Geometry: see drawing. Coordinates: mm, zero at the bounding-box minimum. A direction names the side the tool comes from. Coordinates: 2 decimals unless noted, no trailing zeros. Write each loop counter-clockwise with the first axis right and the second up, starting at its lowest first coordinate (ties: lowest second). Pieces come first, ordered by that corner, then holes.
1) Section query C-C (y = 4). Output: boundary loops of the cut face in (x, z), then the cut area to 3 significant figures.
2) Pin query (flat end, axial travel): pin 1 Ø3 at (x, z) = (13, 1) entering from +Y; pin 2 Ø4 at (x, z) = (36.5, 7) entering from +Y (1 decimal); pin 3 Ø3 at (x, z) = (33.5, 5) entering from -Y; pin 4 Ø1 at (y, z) = (43.5, 5) entering from +X (1 decimal). Return the tip coordinate at first contact, or that it passes through.
3) Section query B-B (z = 6). Output: boundary loops of the cut face in (x, y) (1 decimal).
4) Section query D-D (z = 2). Output: boundary loops of the cut face in (x, y).
5) Line query: L1, parallel to Y at x = 50, z = 7.75 (1 decimal); L2, parallel to X at y = 7.5, z = 7.25 (1 decimal); L3, parallel to Z at x = 31, y = 23.5. Output: solid intervals per line, ascending.
6) Section query A-A (x = 5). Output: boundary loops of the cut face in (y, z).
7) Set-up query: the marked faces 1 and 2. Return all of +Z, -Z, +X, -X, +Y, -Y with unobstructed straight access to the full face (end or side cutting, diameter ignored); none if empty.
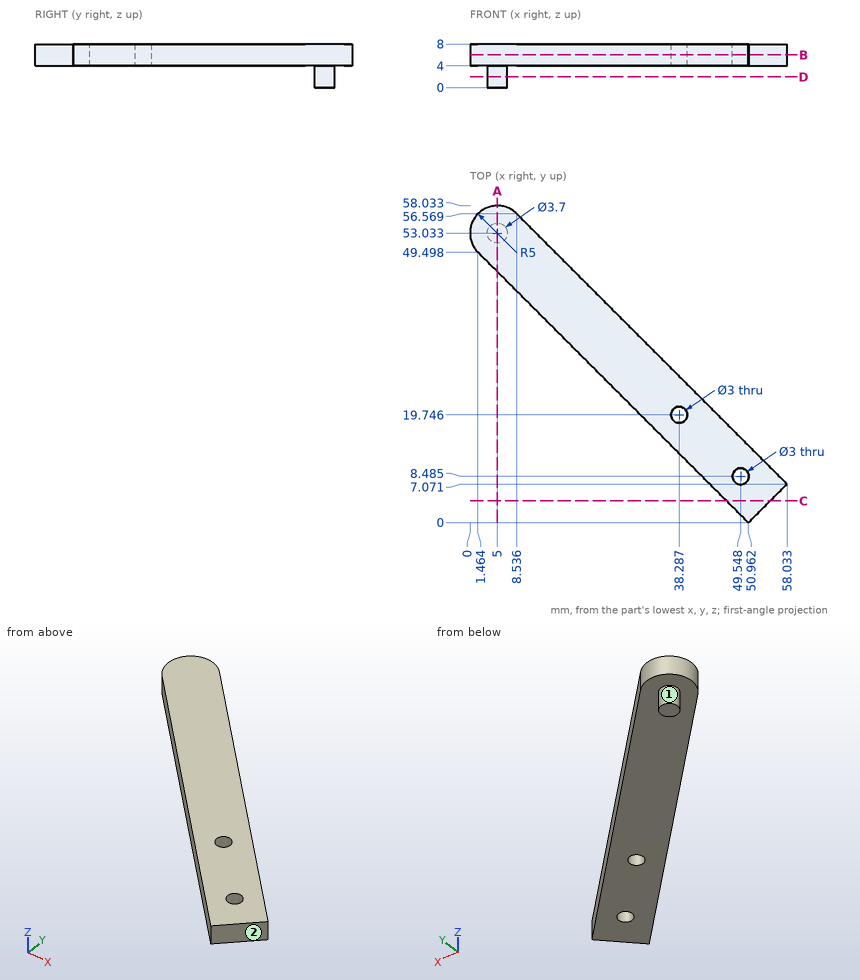
Answer:
1. outline: (46.96, 4) - (54.96, 4) - (54.96, 8) - (46.96, 8) - close
1. area: 32.0 mm2
2. pin 1: passes through
2. pin 2: stops at y = 30.6
2. pin 3: stops at y = 15.96
2. pin 4: stops at x = 22.1
3. outline: (1.5, 49.5) - (51, 0) - (58, 7.1) - (8.5, 56.6) arc R5 ccw to start; hole circle Ø3 at (38.3, 19.7); hole circle Ø3 at (49.5, 8.5)
4. outline: circle Ø3.7 at (5, 53.03)
5. L1: y = 1 to 7.1, 9.9 to 15.1
5. L2: x = 43.5 to 48.4, 50.7 to 57.6
5. L3: z = 4 to 8
6. outline: (45.96, 4) - (51.18, 4) - (51.18, 0) - (54.88, 0) - (54.88, 4) - (58.03, 4) - (58.03, 8) - (45.96, 8) - close
7. face 1: -Z
7. face 2: +Z, -Z, +X, -Y
